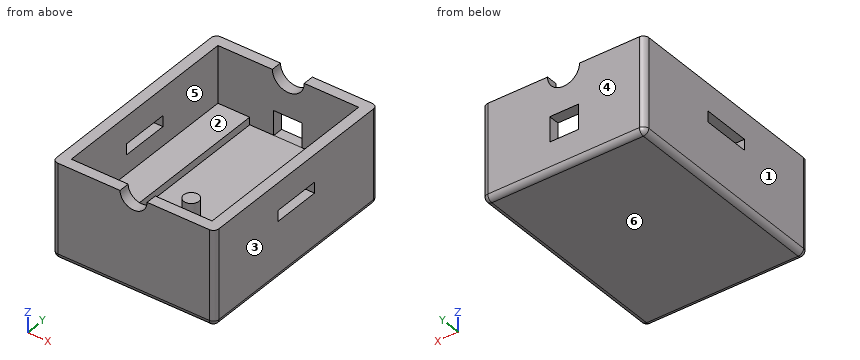
from build123d import *

# Parameters (mm, degrees)
SKETCH1_W               = 30
SKETCH1_H               = 40
BOSS_EXTRUDE1_DEPTH     = 17.5
SKETCH2_W               = 26
SKETCH2_H               = 36
CUT_EXTRUDE1_DEPTH      = 15.5
BOSS_EXTRUDE2_DEPTH     = 3.62
CUT_EXTRUDE5_DEPTH      = 29
CUT_EXTRUDE5_DEPTH_BACK = 3
CUT_EXTRUDE6_DEPTH      = 3
SKETCH13_W              = 5.875
SKETCH13_H              = 36
BOSS_EXTRUDE4_DEPTH     = 5
CUT_EXTRUDE7_REACH      = 42
CUT_EXTRUDE8_DEPTH      = 3
SKETCH16_R              = 1.4
BOSS_EXTRUDE5_DEPTH     = 3.8
FILLET1_R               = 1


with BuildPart() as part:
    # Sketch1 → Boss-Extrude1 (new body)
    with BuildSketch(Plane.XY):
        Rectangle(SKETCH1_W, SKETCH1_H)
    extrude(amount=BOSS_EXTRUDE1_DEPTH)

    # Sketch2 → Cut-Extrude1 (cut)
    with BuildSketch(Plane.XY.offset(17.5)):
        Rectangle(SKETCH2_W, SKETCH2_H)
    extrude(amount=-CUT_EXTRUDE1_DEPTH, mode=Mode.SUBTRACT)

    # Sketch6 → Boss-Extrude2 (add)
    with BuildSketch(Plane.XY.offset(2)):
        Polygon((7.125, 18), (0, 18), (-7.125, 18), (-7.125, -13), (-7.125, -18), (7.125, -18), (7.125, -13), align=None)
    extrude(amount=BOSS_EXTRUDE2_DEPTH)

    # Sketch10 → Cut-Extrude5 (cut, two sides)
    with BuildSketch(Plane.ZY.offset(-13)) as cut_extrude5_sk:
        Polygon((12.5, 0), (12.5, -4.5), (10.5, -4.5), (10.5, 0), (10.5, 4.5), (12.5, 4.5), align=None)
    extrude(amount=CUT_EXTRUDE5_DEPTH, mode=Mode.SUBTRACT)
    extrude(cut_extrude5_sk.sketch, amount=-CUT_EXTRUDE5_DEPTH_BACK, mode=Mode.SUBTRACT)

    # Sketch12 → Cut-Extrude6 (cut, through all)
    with BuildSketch(Plane(origin=(0, -18, 0), x_dir=(1, 0, 0), z_dir=(0, 1, 0))):
        with BuildLine():
            Line((2.5, -17.5), (-2.5, -17.5))
            ThreePointArc((-2.5, -17.5), (0, -15), (2.5, -17.5))
        make_face()
    extrude(amount=-CUT_EXTRUDE6_DEPTH, mode=Mode.SUBTRACT)

    # Sketch13 → Boss-Extrude4 (add)
    with BuildSketch(Plane.XY.offset(2)):
        with Locations((-10.0625, 0)):
            Rectangle(SKETCH13_W, SKETCH13_H)
        with Locations((10.0625, 0)):
            Rectangle(SKETCH13_W, SKETCH13_H)
    extrude(amount=BOSS_EXTRUDE4_DEPTH)

    # Sketch14 → Cut-Extrude7 (cut, up to next)
    with BuildSketch(Plane(origin=(0, 20, 0), x_dir=(1, 0, 0), z_dir=(0, 1, 0)), mode=Mode.PRIVATE) as cut_extrude7_sk1:
        with BuildLine():
            Line((2.95, -17.5), (-2.95, -17.5))
            ThreePointArc((-2.95, -17.5), (0, -14.55), (2.95, -17.5))
        make_face()
    cut_extrude7_tool1 = extrude(cut_extrude7_sk1.sketch, amount=-CUT_EXTRUDE7_REACH, mode=Mode.PRIVATE) & part.part
    add(cut_extrude7_tool1.solids().sort_by_distance((0, 20, 16.247981))[0], mode=Mode.SUBTRACT)

    # Sketch15 → Cut-Extrude8 (cut, through all)
    with BuildSketch(Plane.XZ.offset(-18)):
        Polygon((-2.75, 10.12), (-2.75, 5.52), (2.55, 5.52), (2.55, 7.82), (2.55, 10.12), align=None)
    extrude(amount=-CUT_EXTRUDE8_DEPTH, mode=Mode.SUBTRACT)

    # Sketch16 → Boss-Extrude5 (add)
    with BuildSketch(Plane.XY.offset(5.62)):
        with Locations((0.3, -6.225)):
            Circle(SKETCH16_R)
    extrude(amount=BOSS_EXTRUDE5_DEPTH)

    # Fillet1
    fillet1_edges = [part.edges().sort_by_distance(p)[0] for p in [
        (0, -20, 0),
        (-15, 0, 0),
        (0, 20, 0),
        (15, 0, 0),
        (15, -20, 8.75),
        (-15, -20, 8.75),
        (-15, 20, 8.75),
        (15, 20, 8.75),
    ]]
    fillet(fillet1_edges, radius=FILLET1_R)


solid = part.part
The model under review builds one solid part; all positions refer to its coordinate system, in mm. Face numbers are marked on the shaded views. A direction names the side the tool comes from. Round coordinates to 2 decimals unless told otherwise and drop trailing zeros. Write each loop counter-clockwise with the first axis right and the second up, starting at its lowest first coordinate (ties: lowest second). Pieces come first, ordered by that corner, then holes. Notation, with made-up numbers: M 43,23 L 66,23 A19 cw 66,42 Z; hole C 50,51 d3. An arc over 180 degrees is marked long. Use a Markdown table: item, result. Add a question column.
Q1. We need section A-A, the plane z = 13.5. State the section outline as (x, y) points.
Q2. To check wall thickness, follow line 1 (Y direction, x = 8.75, z = 15); line 2 (X direction, y = -5.5, z = 15.25); line 3 (Z direction, x = 5.5, y = -6.5). State the ranges of each line that lie inside material, in increasing order.
Q3. Machinability: for the marked faces 5 and 6, which of the approach directions +Z, -Z, +X, -X, +Y, -Y give a long, thin tool a straight path to every point of the face, cutting with its end or side? Answer none if there is none.
Q4. We need section C-C, the plane y = 1.5. State the section outline as (x, z) points (3 decimals), plus the area to 3 significant figures.
Q5. We need section D-D, the plane y = -16. State the section outline as (x, z) points (3 decimals).
Q6. Insertion check: pin 1 (0.6 mm diameter, centred on x = -14.5, y = -0.5, fed in from -Z); pin 2 (2 mm diameter, centred on x = -1.5, y = 9, fed in from +Z); pin 3 (4.5 mm diameter, centred on x = 9.5, y = 7.5, fed in from +Z). Each pin has a flat end and moves straight along its axis. Give the tip position at first contact, or say it passes through.
Q7. We need section B-B, the plane x = 0. State the section outline as (y, z) points, plus the area to 3 significant figures.
Q8. The part is to be moulded in two halves that separate along X. For the marked faces 1, 2, 3 and 4, say which applies: pulls with the +X half, pulls with the -X half, needs draft (parallel to the pull), parting line crosses it, or undercut.
Findings below:
| question | item | result |
|---|---|---|
| 1 | outline | M -15,-19 A1 ccw -14,-20 L 14,-20 A1 ccw 15,-19 L 15,19 A1 ccw 14,20 L -14,20 A1 ccw -15,19 Z; hole M -13,-18 L 13,-18 L 13,18 L -13,18 Z |
| 2 | line 1 | y = -20 to -18, 18 to 20 |
| 2 | line 2 | x = -15 to -13, 13 to 15 |
| 2 | line 3 | z = 0 to 5.62 |
| 3 | face 5 | +Z |
| 3 | face 6 | -Z, +X, -X, +Y, -Y |
| 4 | outline | M -15,1 A1 ccw -14,0 L 14,0 A1 ccw 15,1 L 15,10.5 L 13,10.5 L 13,7 L 7.125,7 L 7.125,5.62 L -7.125,5.62 L -7.125,7 L -13,7 L -13,10.5 L -15,10.5 Z; M -15,12.5 L -13,12.5 L -13,17.5 L -15,17.5 Z; M 13,12.5 L 15,12.5 L 15,17.5 L 13,17.5 Z |
| 4 | area | 224 mm² |
| 5 | outline | M -15,1 A1 ccw -14,0 L 14,0 A1 ccw 15,1 L 15,17.5 L 13,17.5 L 13,7 L 7.125,7 L 7.125,5.62 L -7.125,5.62 L -7.125,7 L -13,7 L -13,17.5 L -15,17.5 Z |
| 6 | pin 1 | stops at z = 0.02 |
| 6 | pin 2 | stops at z = 5.62 |
| 6 | pin 3 | stops at z = 7 |
| 7 | outline | M -20,1 A1 ccw -19,0 L 19,0 A1 ccw 20,1 L 20,5.52 L 18,5.52 L 18,5.62 L -4.86,5.62 L -4.86,9.42 L -7.59,9.42 L -7.59,5.62 L -18,5.62 L -18,15 L -20,15 Z; M 18,10.12 L 20,10.12 L 20,14.55 L 18,14.55 Z |
| 7 | area | 262 mm² |
| 8 | face 1 | pulls with the -X half |
| 8 | face 2 | undercut |
| 8 | face 3 | pulls with the +X half |
| 8 | face 4 | needs draft |
